The listing builds one solid part. Answer for the finished solid, in the listing's coordinates (mm). Give positions to 0.01 mm unless a question says otherwise; leave off trailing zeros. Write each loop counter-clockwise with the first axis right and the second up, starting at its lowest first coordinate (ties: lowest second). Pieces come first, ordered by that corner, then holes. Notation, with made-up numbers: (53.25, 58) -> (95.25, 58) arc R17 ccw to (95.25, 68) -> close; hole circle Ø5 at (-28.75, 27.5). An arc over 180 degrees is marked (long way). Put each result on its own line as item: value. Start each with the question number.
1) A cutting plane is placed at A-A (z = 13). Write down the section's boundary in (x, y).
2) A cutting plane is placed at C-C (y = 737). Write down the section's boundary in (x, z).
3) Find the intervals of material crossed by line 1 along X through (y, z) = (792, 24.25); line 2 along X through (y, z) = (424, 9.75); line 3 along Y through (x, z) = (-616, 20), in increasing order. Write a range as from..to.
4) A cutting plane is placed at B-B (y = 291.5). Write down the section's boundary in (x, z), then the cut area to 3 significant figures.
from build123d import *

# Parameters (mm, degrees)
F1_DEPTH = 25.4


with BuildPart() as f1:
    # F0 (on Top) → F1 (new body)
    with BuildSketch(Plane.XY):
        with BuildLine():
            Line((-1063.343933, 1044.720739), (-1495.143933, 1044.720739))
            Line((-1495.143933, 1044.720739), (-1495.143933, 511.320739))
            Line((-1495.143933, 511.320739), (-1114.143933, 511.320739))
            ThreePointArc((-1114.143933, 511.320739), (-1101.224902, 609.694516), (-1063.343933, 701.396934))
            Line((-1063.343933, 701.396934), (-1063.343933, 1044.720739))
        make_face()
        with BuildLine():
            Line((-733.143933, 1044.720739), (-1063.343933, 1044.720739))
            Line((-1063.343933, 1044.720739), (-1063.343933, 701.396934))
            ThreePointArc((-1063.343933, 701.396934), (-923.855718, 841.154053), (-733.143933, 892.320739))
            Line((-733.143933, 892.320739), (-733.143933, 1044.720739))
        make_face()
        with BuildLine():
            Line((-1114.143933, 511.320739), (-1495.143933, 511.320739))
            Line((-1495.143933, 511.320739), (-1495.143933, -22.079261))
            Line((-1495.143933, -22.079261), (-1063.343933, -22.079261))
            Line((-1063.343933, -22.079261), (-1063.343933, 321.244544))
            ThreePointArc((-1063.343933, 321.244544), (-1101.224902, 412.946962), (-1114.143933, 511.320739))
        make_face()
        with BuildLine():
            Line((-402.943933, 1044.720739), (-733.143933, 1044.720739))
            Line((-733.143933, 1044.720739), (-733.143933, 892.320739))
            ThreePointArc((-733.143933, 892.320739), (-542.432148, 841.154053), (-402.943933, 701.396934))
            Line((-402.943933, 701.396934), (-402.943933, 1044.720739))
        make_face()
        with BuildLine():
            Line((28.856067, 1044.720739), (-402.943933, 1044.720739))
            Line((-402.943933, 1044.720739), (-402.943933, 701.396934))
            ThreePointArc((-402.943933, 701.396934), (-365.062964, 609.694516), (-352.143933, 511.320739))
            Line((-352.143933, 511.320739), (28.856067, 511.320739))
            Line((28.856067, 511.320739), (28.856067, 1044.720739))
        make_face()
        with BuildLine():
            Line((-1063.343933, 321.244544), (-1063.343933, -22.079261))
            Line((-1063.343933, -22.079261), (-733.143933, -22.079261))
            Line((-733.143933, -22.079261), (-733.143933, 130.320739))
            ThreePointArc((-733.143933, 130.320739), (-923.855718, 181.487425), (-1063.343933, 321.244544))
        make_face()
        with BuildLine():
            Line((-733.143933, 130.320739), (-733.143933, -22.079261))
            Line((-733.143933, -22.079261), (-402.943933, -22.079261))
            Line((-402.943933, -22.079261), (-402.943933, 321.244544))
            ThreePointArc((-402.943933, 321.244544), (-542.432148, 181.487425), (-733.143933, 130.320739))
        make_face()
        with BuildLine():
            Line((28.856067, -22.079261), (28.856067, 511.320739))
            Line((28.856067, 511.320739), (-352.143933, 511.320739))
            ThreePointArc((-352.143933, 511.320739), (-365.062964, 412.946962), (-402.943933, 321.244544))
            Line((-402.943933, 321.244544), (-402.943933, -22.079261))
            Line((-402.943933, -22.079261), (28.856067, -22.079261))
        make_face()
    extrude(amount=F1_DEPTH)


solid = f1.part
Reply:
1. outline: (-1495.14, -22.08) -> (28.86, -22.08) -> (28.86, 1044.72) -> (-1495.14, 1044.72) -> close; hole (-1114.14, 511.32) arc R381 ccw to (-1063.34, 321.24) arc R381 ccw to (-402.94, 321.24) arc R381 ccw to (-352.14, 511.32) arc R381 ccw to (-402.94, 701.4) arc R381 ccw to (-1063.34, 701.4) arc R381 ccw to start
2. outline: (-1495.14, 0) -> (-1040.11, 0) -> (-1040.11, 25.4) -> (-1495.14, 25.4) -> close; (-426.18, 0) -> (28.86, 0) -> (28.86, 25.4) -> (-426.18, 25.4) -> close
3. line 1: x = -1495.14..-990.79, -475.5..28.86
3. line 2: x = -1495.14..-1104, -362.29..28.86
3. line 3: y = -22.08..148.78, 873.86..1044.72
4. outline: (-1495.14, 0) -> (-1044.33, 0) -> (-1044.33, 25.4) -> (-1495.14, 25.4) -> close; (-421.95, 0) -> (28.86, 0) -> (28.86, 25.4) -> (-421.95, 25.4) -> close
4. area: 22,900 mm2
